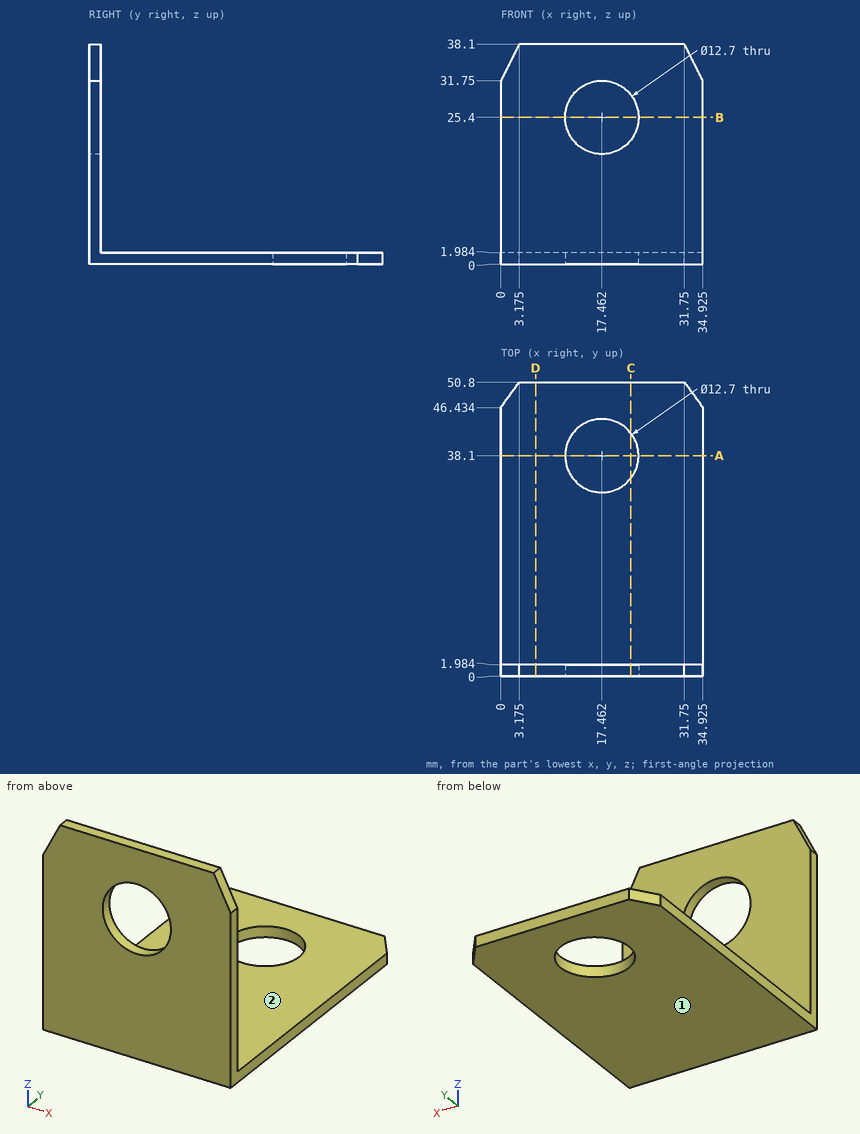
Input: dimensioned drawing with shaded views. Units: mm. Origin: part minimum x, y, z. A direction names the side the tool comes from. Round coordinates to 2 decimals unless told otherwise and drop trailing zeros. Write each loop counter-clockwise with the first axis right and the second up, starting at its lowest first coordinate (ties: lowest second). Pieces come first, ordered by that corner, then holes. Notation, with made-up numbers: (81, 31.5) -> (89, 31.5) arc R17 ccw to (89, 61.5) -> close; hole circle Ø9 at (12.25, 47.25). An arc over 180 degrees is marked (long way). Use CSV: the item, a comma, the result in double quotes. Start each with the question number.
Q1. Line query: L1, parallel to X at y = 1.15, z = 25.4 (1 decimal); L2, parallel to Z at x = 30, y = 13 (1 decimal). Output: solid intervals per line, ascending.
Q2. Section D-D (x = 6). Return loops of the section in (y, z) (1 decimal).
Q3. Reachability of the marked faces 1 and 2 from +Z, -Z, +X, -X, +Y, -Y: full face, straight path, thin tool, end or side. Return the list, or none.
Q4. First-contact query: pin 1 Ø6 at (x, y) = (6.5, 44.5) entering from +Z; pin 2 Ø12 at (y, z) = (16, 10.5) entering from -X; pin 3 Ø10 at (x, z) = (24, 24) entering from +Y. Flat tips, straight axial feed; report the tip coordinate or a pass-through.
Q5. Section A-A (y = 38.1). Return loops of the section in (x, z) (1 decimal).
Q6. Section C-C (x = 22.5). Return loops of the section in (y, z) (1 decimal).
Result sheet:
1,L1,"0 to 11.1, 23.8 to 34.9"
1,L2,"0 to 2"
2,outline,"(0, 0) -> (50.8, 0) -> (50.8, 2) -> (2, 2) -> (2, 38.1) -> (0, 38.1) -> close"
3,face 1,"-Z, +X, -X, +Y, -Y"
3,face 2,"+Z, +X, -X, +Y"
4,pin 1,"z = 1.98"
4,pin 2,"through"
4,pin 3,"y = 1.98"
5,outline,"(0, 0) -> (11.1, 0) -> (11.1, 2) -> (0, 2) -> close; (23.8, 0) -> (34.9, 0) -> (34.9, 2) -> (23.8, 2) -> close"
6,outline,"(0, 0) -> (34.2, 0) -> (34.2, 2) -> (2, 2) -> (2, 21.5) -> (0, 21.5) -> close; (0, 29.3) -> (2, 29.3) -> (2, 38.1) -> (0, 38.1) -> close; (42, 0) -> (50.8, 0) -> (50.8, 2) -> (42, 2) -> close"
